from build123d import *

# Parameters (mm, degrees)
BOSS_EXTRUDE1_DEPTH            = 171.45
FILLET1_R                      = 2.955
TAP_DRILL_FOR_10_32_TAP1_D     = 4.0386
TAP_DRILL_FOR_10_32_TAP1_DEPTH = 12.7
TAP_DRILL_FOR_10_32_TAP1_TIP   = 1.213317848
TAP_DRILL_FOR_10_32_TAP2_D     = 4.0386
TAP_DRILL_FOR_10_32_TAP2_DEPTH = 12.7
TAP_DRILL_FOR_10_32_TAP2_TIP   = 1.213317848
SKETCH12_OUTSIDE_W             = 49.194
SKETCH12_OUTSIDE_H             = 50.244
SKETCH12_OUTSIDE_R             = 6.35
CUT_EXTRUDE2_DEPTH             = 120.65
CUT_EXTRUDE3_DEPTH             = 1.9177


with BuildPart() as part:
    # Sketch3 → Boss-Extrude1 (new body)
    with BuildSketch(Plane.XY):
        Polygon((0, 7.332348419), (-6.35, 3.666174209), (-6.35, -3.666174209), (0, -7.332348419), (6.35, -3.666174209), (6.35, 3.666174209), align=None)
    extrude(amount=BOSS_EXTRUDE1_DEPTH)

    # Fillet1
    fillet1_edges = [part.edges().sort_by_distance(p)[0] for p in [
        (6.35, 3.666174209, 85.725),
        (6.35, -3.666174209, 85.725),
        (0, -7.332348419, 85.725),
        (-6.35, -3.666174209, 85.725),
        (-6.35, 3.666174209, 85.725),
        (0, 7.332348419, 85.725),
    ]]
    fillet(fillet1_edges, radius=FILLET1_R)

    # Tap Drill for #10-32 Tap1
    with Locations(Plane(origin=(0, 0, 0), x_dir=(-1, 0, 0), z_dir=(0, 0, -1))):
        with Locations((0, 0)):
            Hole(TAP_DRILL_FOR_10_32_TAP1_D / 2, depth=TAP_DRILL_FOR_10_32_TAP1_DEPTH)
            with Locations((0, 0, -(TAP_DRILL_FOR_10_32_TAP1_DEPTH + TAP_DRILL_FOR_10_32_TAP1_TIP / 2))):  # 118° drill point
                Cone(0, TAP_DRILL_FOR_10_32_TAP1_D / 2, TAP_DRILL_FOR_10_32_TAP1_TIP, mode=Mode.SUBTRACT)

    # Tap Drill for #10-32 Tap2
    with Locations(Plane.XY.offset(171.45)):
        with Locations((0, 0)):
            Hole(TAP_DRILL_FOR_10_32_TAP2_D / 2, depth=TAP_DRILL_FOR_10_32_TAP2_DEPTH)
            with Locations((0, 0, -(TAP_DRILL_FOR_10_32_TAP2_DEPTH + TAP_DRILL_FOR_10_32_TAP2_TIP / 2))):  # 118° drill point
                Cone(0, TAP_DRILL_FOR_10_32_TAP2_D / 2, TAP_DRILL_FOR_10_32_TAP2_TIP, mode=Mode.SUBTRACT)

    # Sketch12 outside → Cut-Extrude2 (cut)
    with BuildSketch(Plane(origin=(0, 0, 0), x_dir=(-1, 0, 0), z_dir=(0, 0, -1))):
        Rectangle(SKETCH12_OUTSIDE_W, SKETCH12_OUTSIDE_H)
        Circle(SKETCH12_OUTSIDE_R, mode=Mode.SUBTRACT)
    extrude(amount=-CUT_EXTRUDE2_DEPTH, mode=Mode.SUBTRACT)

    # Sketch13 → Cut-Extrude3 (cut)
    with BuildSketch(Plane(origin=(5.61125, 3.239656698, 0), x_dir=(0, 0, 1), z_dir=(-0.866025404, -0.5, 0))):
        with BuildLine():
            Line((92.075, 1.5875), (47.625, 1.5875))
            ThreePointArc((47.625, 1.5875), (46.0375, 0), (47.625, -1.5875))
            Line((47.625, -1.5875), (92.075, -1.5875))
            ThreePointArc((92.075, -1.5875), (93.6625, 0), (92.075, 1.5875))
        make_face()
    extrude(amount=CUT_EXTRUDE3_DEPTH, mode=Mode.SUBTRACT)


solid = part.part
Could you check a few things on this model? Use its own coordinates, in mm. A direction names the side the tool comes from. Give positions to 0.01 mm unless a question says otherwise; leave off trailing zeros. Order: outer loops, then holes, each group sorted by start corner. A loop starts at its lowest first (then second) coordinate and runs counter-clockwise, first axis right, second up.
Item 1: If we mould it in two halves opening along Z, with no side actions, what happens to faces 6 (the face through (-3.199, -5.486, 145.694)), 7 (the face through (4.755, 2.705, 93.662)), 8 (the face through (6, -3, 120.65)), 9 (the face through (3.94, 2.3, 69.52))? For each: pulls with the +Z half, pulls with the -Z half, needs draft (parallel to the pull), parting line crosses it, or undercut.
Item 2: For faces 1 (the face through (6, 3, 120.65)), 2 (the face through (-1.926, 0.607, 165.011)), 3 (the face through (-6, 3, 120.65)), 4 (the face through (-6, -3, 120.65)), 5 (the face through (1.926, 0.607, 6.439)), which set-ups out of +Z, -Z, +X, -X, +Y, -Y let a thin tool reach every point of the face, with its end or its side?
Item 3: I'm going to push flat-ended pins straight in: pin 1 (5 mm diameter, centred on x = 1, z = 37.5, fed in from -Y); pin 2 (3 mm diameter, centred on x = 2, z = 79.5, fed in from +Y); pin 3 (1.5 mm diameter, centred on x = 4, z = 123.5, fed in from +Y). Where does each tip first touch, or does it pass through?
Item 4: I need wall thicknesses on line 1 (Y direction, x = 0, z = 9.75); line 2 (Y direction, x = 0, z = 167). Which ranges of each line are inside material? Lowest first, please.
Item 5: If we section it at B-B, the plane z = 64: Write out the boundary of the cut face in (x, y).
Item 6: If we section it at C-C, the plane z = 36: Write out the boundary of the cut face in (x, y), plus the area to 3 significant figures.
Values:
1. face 6: needs draft
1. face 7: undercut
1. face 8: pulls with the -Z half
1. face 9: undercut
2. face 1: -Z, +X, +Y
2. face 2: +Z
2. face 3: -Z, -X, +Y
2. face 4: -Z, -X, -Y
2. face 5: -Z
3. pin 1: stops at y = -6.35
3. pin 2: stops at y = 6.33
3. pin 3: stops at y = 5.46
4. line 1: y = -6.35 to -2.02, 2.02 to 6.35
4. line 2: y = -6.88 to -2.02, 2.02 to 6.88
5. outline: (3.16, 3.66) - (4.53, 4.45) arc R6.35 ccw (long way) to (6.12, 1.7) - (4.74, 0.91) - close
6. outline: circle Ø12.7 at (0, 0)
6. area: 127 mm2
